Could you check a few things on this drawing? It's one solid part, dimensions in mm from its lowest x, y, z. Give positions to 0.01 mm unless a question says otherwise; leave off trailing zeros. Loops run counter-clockwise (first coordinate to the right, second up) from the corner with the lowest first, then second, coordinate; pieces in that order, holes last. Notation, with made-up numbers: M -30,8.5 L -22,8.5 A10 ccw -22,17.5 Z; hole C 89,72.5 d6. An arc over 180 degrees is marked long. Answer as a JSON object with one key per item and string values.
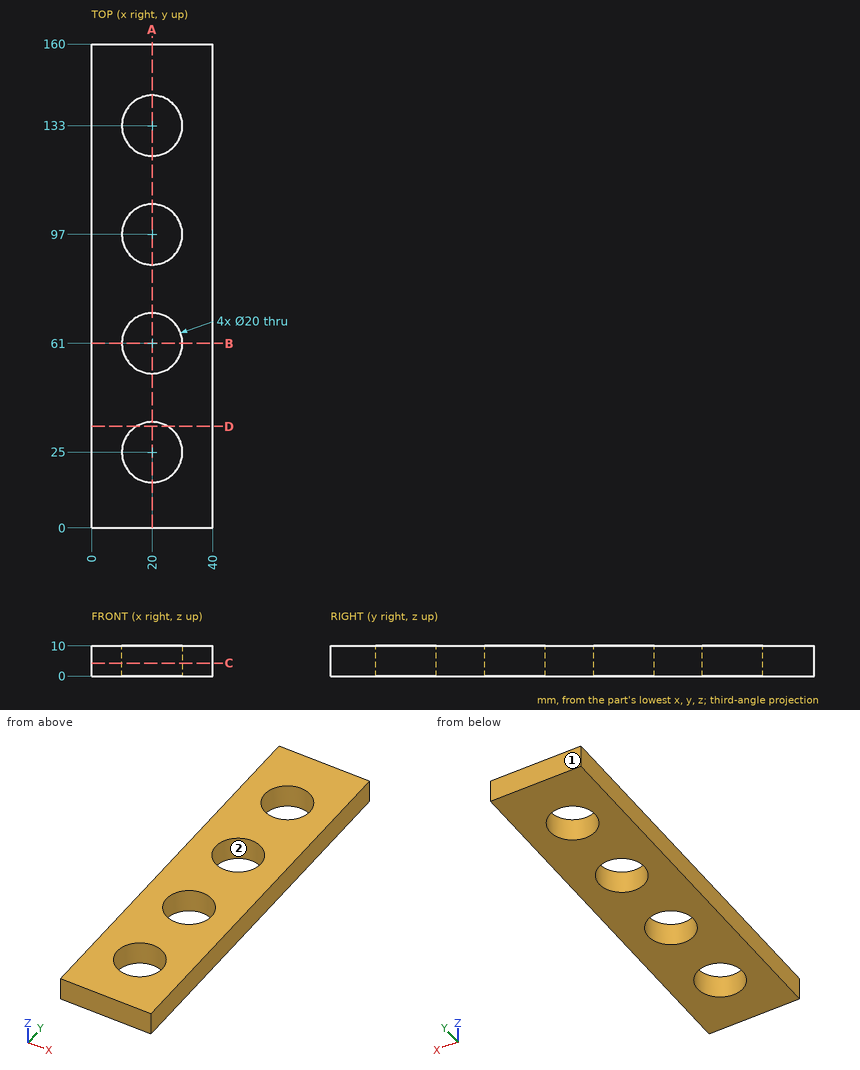
1) Please list where these lines run through material, in increasing order: line 1 along Y through (x, z) = (20, 8.25); line 2 along Y through (x, z) = (11.5, 7.5); line 3 along X through (y, z) = (18, 1.25). Write a range as from..to.
Answer list:
{"line 1": "0..15, 35..51, 71..87, 107..123, 143..160", "line 2": "0..19.73, 30.27..55.73, 66.27..91.73, 102.27..127.73, 138.27..160", "line 3": "0..12.86, 27.14..40"}
2) If we mould it in two halves opening along X, with no side actions, what happens to the marked faces 1 and 2? For each: +X half, -X half, draft (parallel to the pull), parting line (faces both ways), or undercut.
Answer list:
{"face 1": "draft", "face 2": "undercut"}
3) Suppose I cut it at C-C, the plane z = 4.25. Write out the boundary of the cut face in (x, y).
Answer list:
{"outline": "M 0,0 L 40,0 L 40,160 L 0,160 Z; hole C 20,25 d20; hole C 20,61 d20; hole C 20,97 d20; hole C 20,133 d20"}
4) Suppose I cut it at A-A, the plane x = 20. Write out the boundary of the cut face in (y, z).
Answer list:
{"outline": "M 0,0 L 15,0 L 15,10 L 0,10 Z; M 35,0 L 51,0 L 51,10 L 35,10 Z; M 71,0 L 87,0 L 87,10 L 71,10 Z; M 107,0 L 123,0 L 123,10 L 107,10 Z; M 143,0 L 160,0 L 160,10 L 143,10 Z"}
5) Suppose I cut it at D-D, the plane y = 33.5. Write out the boundary of the cut face in (x, z).
Answer list:
{"outline": "M 0,0 L 14.73,0 L 14.73,10 L 0,10 Z; M 25.27,0 L 40,0 L 40,10 L 25.27,10 Z"}
6) Suppose I cut it at B-B, the plane y = 61. Write out the boundary of the cut face in (x, z), and give its area (3 significant figures).
Answer list:
{"outline": "M 0,0 L 10,0 L 10,10 L 0,10 Z; M 30,0 L 40,0 L 40,10 L 30,10 Z", "area": "200 mm^2"}
